from build123d import *

# Parameters (mm, degrees)
F0_W        = 70
F0_H        = 45
F1_DEPTH    = 25
F2_T        = -2.5
F3_T1_DEPTH = 40
F3_T3_DEPTH = 65
F4_SIZE     = 4
F5_SIZE     = 1.5


# Not quite as in the source:
# - a fillet or chamfer that OpenCascade refuses, or shapes differently, is made with other operations: its cross-section is extruded or revolved along the edge and cut away or added


with BuildPart() as f1:
    # F0 (on Top) → F1 (new body)
    with BuildSketch(Plane.XY):
        with Locations((9.3095207959, -39.4999814034)):
            Rectangle(F0_W, F0_H)
    extrude(amount=F1_DEPTH)

    # F2
    f2_openings = [f1.faces().sort_by_distance(p)[0] for p in [
        (9.309521, -39.499981, 25),
    ]]
    offset(amount=F2_T, openings=f2_openings)

    # F3: fillet of radius 5 on 4 edges, made by hand

    # F3_s2 → F3_t1 (join)
    with BuildSketch(Plane.XZ.offset(19.4999814034)):
        with BuildLine():
            add(Edge.make_bspline(
                [(-23.1904792041, 7.5), (-23.1904792041, 2.5), (-18.1904792041, 2.5)],
                knots=[0, 0, 0, 1, 1, 1], degree=2, weights=[1, 1, 1]))
            Line((-18.1904792041, 2.5), (-23.1904792041, 2.5))
            Line((-23.1904792041, 2.5), (-23.1904792041, 7.5))
        make_face()
        with BuildLine():
            add(Edge.make_bspline(
                [(41.8095207959, 7.5), (41.8095207959, 2.5), (36.8095207959, 2.5)],
                knots=[0, 0, 0, 1, 1, 1], degree=2, weights=[1, 1, 1]))
            Line((36.8095207959, 2.5), (41.8095207959, 2.5))
            Line((41.8095207959, 2.5), (41.8095207959, 7.5))
        make_face()
    extrude(amount=F3_T1_DEPTH)

    # F3_s4 → F3_t3 (join)
    with BuildSketch(Plane.YZ.offset(-23.1904792041)):
        with BuildLine():
            add(Edge.make_bspline(
                [(-19.4999814034, 7.5), (-19.4999814034, 2.5), (-24.4999814034, 2.5)],
                knots=[0, 0, 0, 1, 1, 1], degree=2, weights=[1, 1, 1]))
            Line((-24.4999814034, 2.5), (-19.4999814034, 2.5))
            Line((-19.4999814034, 2.5), (-19.4999814034, 7.5))
        make_face()
        with BuildLine():
            add(Edge.make_bspline(
                [(-59.4999814034, 7.5), (-59.4999814034, 2.5), (-54.4999814034, 2.5)],
                knots=[0, 0, 0, 1, 1, 1], degree=2, weights=[1, 1, 1]))
            Line((-54.4999814034, 2.5), (-59.4999814034, 2.5))
            Line((-59.4999814034, 2.5), (-59.4999814034, 7.5))
        make_face()
    extrude(amount=F3_T3_DEPTH)

    # F4
    f4_edges = [f1.edges().sort_by_distance(p)[0] for p in [
        (9.309521, -61.999981, 0),
        (-25.690479, -39.499981, 0),
        (44.309521, -39.499981, 0),
        (9.309521, -16.999981, 0),
    ]]
    chamfer(f4_edges, length=F4_SIZE)

    # F5
    f5_edges = [f1.edges().sort_by_distance(p)[0] for p in [
        (9.309521, -19.499981, 25),
        (-23.190479, -39.499981, 25),
        (9.309521, -59.499981, 25),
        (41.809521, -39.499981, 25),
    ]]
    chamfer(f5_edges, length=F5_SIZE)


solid = f1.part
For this review, take the finished solid that the model builds, in its own axes (mm). A direction names the side the tool comes from. Round coordinates to 2 decimals unless told otherwise and drop trailing zeros. Order: outer loops, then holes, each group sorted by start corner. A loop starts at its lowest first (then second) coordinate and runs counter-clockwise, first axis right, second up. Notation, with made-up numbers: (-10, 16.5) -> (1, 16.5) arc R14 ccw to (1, 37.5) -> close; hole circle Ø10 at (51, 27.25). An arc over 180 degrees is marked (long way). Put each result on its own line as item: value.
Q1. Insertion check: pin 1 Ø1 at (x, y) = (29, -49) entering from +Z; pin 2 Ø24 at (x, y) = (-4.5, -33) entering from +Z. Each pin has a flat end and moves straight along its axis. Give the tip position at first contact, or say it passes through.
Check result:
pin 1: z = 2.5
pin 2: z = 3.52
Q2. Add section A-A on z = 15.5. Write out the cut boundary in (x, y).
Check result:
outline: (-25.69, -62) -> (44.31, -62) -> (44.31, -17) -> (-25.69, -17) -> close; hole (-23.19, -59.5) -> (41.81, -59.5) -> (41.81, -19.5) -> (-23.19, -19.5) -> close
Q3. Mouldability with a two-part tool opening along X and no side actions: class faces 3 (the flat face through (9, -39, 2.5)), 4 (the flat face through (-25.69, -40, 14)), 5 (the flat face through (9, -19, 24)), 6 (the flat face through (9, -60, 2)) as pulls with the +X half, pulls with the -X half, needs draft (parallel to the pull), parting line crosses it, or undercut.
Check result:
face 3: undercut
face 4: pulls with the -X half
face 5: undercut
face 6: needs draft
Q4. Machinability: for faces 1 (the flat face through (9, -19.5, 15)), 2 (the flat face through (9, -39, 0)), which of the approach directions +Z, -Z, +X, -X, +Y, -Y give a long, thin tool a straight path to every point of the face, cutting with its end or side? Answer none if there is none.
Check result:
face 1: +Z
face 2: -Z, +X, -X, +Y, -Y
Q5. For probe 1 along X at (y, z) = (-50.5, 17.75); probe 2 along Y at (x, z) = (13.5, 9.5); probe 3 along Z at (x, y) = (32.5, -50.5), list the stretches that pass through material, from the lowest coordinate up. Write a range as [from, to].
Check result:
probe 1: [-25.69, -23.19], [41.81, 44.31]
probe 2: [-62, -59.5], [-19.5, -17]
probe 3: [0, 2.5]
